from build123d import *

# Parameters (mm, degrees)
F1_DEPTH = 63.5
F2_DEPTH = 25.4
F3_DEPTH = 7.9375
F5_R     = 6.35


# Not quite as in the source:
# - a feature names something its author has since deleted; it is built from what else it names


with BuildPart() as f1:
    # F0 (on Front) → F1 (new body, symmetric)
    with BuildSketch(Plane.XZ):
        Polygon((41.275, -9.525), (41.275, 9.525), (22.225, 9.525), (-41.275, 9.525), (-41.275, -9.525), align=None)
    extrude(amount=F1_DEPTH, both=True)

    # F0 (on Front) → F2 (join, symmetric)
    with BuildSketch(Plane.XZ):
        with BuildLine():
            Line((22.225, 9.525), (41.275, 9.525))
            Line((41.275, 9.525), (41.275, 27.0002))
            ThreePointArc((41.275, 27.0002), (45.9246798487, 38.2255201513), (57.15, 42.8752))
            Line((57.15, 42.8752), (60.325, 42.8752))
            Line((60.325, 42.8752), (60.325, 61.9252))
            Line((60.325, 61.9252), (57.15, 61.9252))
            add(Edge.make_bspline(
                [(55.3844542669, 61.8805450852), (55.9790813374, 61.8982519362), (56.5677127817, 61.9131134827), (57.15, 61.9252)],
                knots=[109.7272835167, 109.7272835167, 109.7272835167, 109.7272835167, 111.5045361635, 111.5045361635, 111.5045361635, 111.5045361635], degree=3))
            ThreePointArc((55.3844542669, 61.8805450852), (31.8377765721, 51.0635948173), (22.225, 27.0002))
            Line((22.225, 27.0002), (22.225, 9.525))
        make_face()
        Polygon((60.325, 61.9252), (60.325, 42.8752), (71.4375, 42.8752), (85.725, 42.8752), (85.725, 61.9252), (71.4375, 61.9252), align=None)
    extrude(amount=F2_DEPTH, both=True)

    # F0 (on Front) → F3 (join, symmetric)
    with BuildSketch(Plane.XZ):
        with BuildLine():
            Line((-41.275, 9.525), (22.225, 9.525))
            Line((22.225, 9.525), (22.225, 27.0002))
            ThreePointArc((22.225, 27.0002), (31.8377765721, 51.0635948173), (55.3844542669, 61.8805450852))
            add(Edge.make_bspline(
                [(-41.275, 9.525), (-40.8940696255, 48.8483570296), (18.6722776014, 60.7873270442), (55.3844542669, 61.8805450852)],
                knots=[0, 0, 0, 0, 109.7272835167, 109.7272835167, 109.7272835167, 109.7272835167], degree=3))
        make_face()
    extrude(amount=F3_DEPTH, both=True)

    # F0 (on Front) → F4 (revolve)
    with BuildSketch(Plane.XZ):
        Polygon((85.725, 42.8752), (85.725, 38.1), (111.125, 38.1), (111.125, 66.675), (85.725, 66.675), (85.725, 61.9252), align=None)
    revolve(axis=Axis((85.725, 0, 52.4002), (0, 0, 1)))

    # F5
    f5_edges = [f1.edges().sort_by_distance(p)[0] for p in [
        (-41.275, -63.5, 0),
        (41.275, -63.5, 0),
        (41.275, 63.5, 0),
        (-41.275, 63.5, 0),
    ]]
    fillet(f5_edges, radius=F5_R)


solid = f1.part
Source: CAD feature listing. Evaluate the final solid. Frame: model axes, mm. A direction names the side the tool comes from. Coordinates: 2 decimals unless noted, no trailing zeros. Loops run counter-clockwise (first coordinate to the right, second up) from the corner with the lowest first, then second, coordinate; pieces in that order, holes last. Notation, with made-up numbers: M 47.25,71 L 81.25,71 A17 cw 81.25,95 Z; hole C 30,86 d10. An arc over 180 degrees is marked long. Answer in a Markdown table with one row per item.
Q1. Draft query along Y for faces 4 (the cylindrical face through (32.095, -16.791, 51.332)), 5 (the flat face through (-4, -7.938, 30)), 6 (the flat face through (-4, 7.938, 30)). Return one class per face: pulls with the +Y half, pulls with the -Y half, needs draft (parallel to the pull), parting line crosses it, or undercut.
Answers below:
| item | result |
|---|---|
| face 4 | needs draft |
| face 5 | pulls with the -Y half |
| face 6 | pulls with the +Y half |
Q2. Section B-B on x = 69. Return the cut outline in (y, z) (3 decimals), plus the area to 3 significant figures.
Answers below:
| item | result |
|---|---|
| outline | M -25.4,42.875 L -19.116,42.875 L -19.116,38.1 L 19.116,38.1 L 19.116,42.875 L 25.4,42.875 L 25.4,61.925 L 19.116,61.925 L 19.116,66.675 L -19.116,66.675 L -19.116,61.925 L -25.4,61.925 Z |
| area | 1,330 mm^2 |
Q3. First-contact query: pin 1 (6 mm diameter, centred on x = 34, z = 28.5, fed in from +Y); pin 2 (2 mm diameter, centred on x = -16, z = 16, fed in from -Y); pin 3 (15.5 mm diameter, centred on x = 57.5, z = 40.5, fed in from -Y). Flat tips, straight axial feed; report the tip coordinate or a pass-through.
Answers below:
| item | result |
|---|---|
| pin 1 | stops at y = 25.4 |
| pin 2 | stops at y = -7.94 |
| pin 3 | stops at y = -25.4 |
Q4. Ray query, probe 1 along X at (y, z) = (7, 5) (3 decimals); probe 2 along Z at (x, y) = (34.5, 43) (3 decimals); probe 3 along Y at (x, z) = (39, 34). Return the intervals inside material, ascending. Write a range as from..to.
Answers below:
| item | result |
|---|---|
| probe 1 | x = -41.275..41.275 |
| probe 2 | z = -9.525..9.525 |
| probe 3 | y = -25.4..25.4 |
Q5. Section C-C on y = 45. Return the cut outline in (x, z) (3 decimals).
Answers below:
| item | result |
|---|---|
| outline | M -41.275,-9.525 L 41.275,-9.525 L 41.275,9.525 L -41.275,9.525 Z |
Q6. Set-up query: faces 1 (the flat face through (22.225, -17, 18)), 2 (the flat face through (46, 25.4, 42)), 3 (the flat face through (60, -2, 61.925)). Return all of +Z, -Z, +X, -X, +Y, -Y with unobstructed straight access to the full face (end or side cutting, diameter ignored); none if empty.
Answers below:
| item | result |
|---|---|
| face 1 | +Z, -X, -Y |
| face 2 | +Z, +X, -X, +Y |
| face 3 | +Z, -X |
Q7. Section A-A on z = 2.5. Return the cut outline in (x, y) (3 decimals), plus the area to 3 significant figures.
Answers below:
| item | result |
|---|---|
| outline | M -41.275,-57.15 A6.35 ccw -34.925,-63.5 L 34.925,-63.5 A6.35 ccw 41.275,-57.15 L 41.275,57.15 A6.35 ccw 34.925,63.5 L -34.925,63.5 A6.35 ccw -41.275,57.15 Z |
| area | 10,400 mm^2 |
